Read the model definition and answer for the solid it produces. Units are mm, in the model's axes. Coordinates: 2 decimals unless noted, no trailing zeros. Order: outer loops, then holes, each group sorted by start corner. A loop starts at its lowest first (then second) coordinate and runs counter-clockwise, first axis right, second up.
```python
from build123d import *

# Parameters (mm, degrees)
SKETCH1_W           = 11.5
SKETCH1_H           = 11.5
BOSS_EXTRUDE1_DEPTH = 2
SKETCH2_R           = 2
CUT_EXTRUDE1_DEPTH  = 3
FILLET1_R           = 1
FILLET2_R           = 0.5
FILLET3_R           = 0.5


with BuildPart() as part:
    # Sketch1 → Boss-Extrude1 (new body)
    with BuildSketch(Plane(origin=(0, 0, 0), x_dir=(1, 0, 0), z_dir=(0, 1, 0))):
        Rectangle(SKETCH1_W, SKETCH1_H)
    extrude(amount=BOSS_EXTRUDE1_DEPTH)

    # Sketch2 → Cut-Extrude1 (cut, through all)
    with BuildSketch(Plane(origin=(0, 2, 0), x_dir=(1, 0, 0), z_dir=(0, 1, 0))):
        Circle(SKETCH2_R)
    extrude(amount=-CUT_EXTRUDE1_DEPTH, mode=Mode.SUBTRACT)

    # Fillet1
    fillet1_edges = [part.edges().sort_by_distance(p)[0] for p in [
        (0, 2, 5.75),
    ]]
    fillet(fillet1_edges, radius=FILLET1_R)

    # Fillet2
    fillet2_edges = [part.edges().sort_by_distance(p)[0] for p in [
        (0, 2, -5.75),
    ]]
    fillet(fillet2_edges, radius=FILLET2_R)

    # Fillet3
    fillet3_edges = [part.edges().sort_by_distance(p)[0] for p in [
        (-2, 2, 0),
    ]]
    fillet(fillet3_edges, radius=FILLET3_R)


solid = part.part
```
1) A cutting plane is placed at C-C, the plane y = 1.2. Determine the outline of the cut face in (x, z), and give its area (3 significant figures).
A:
outline: (-5.75, -5.75) - (5.75, -5.75) - (5.75, 5.73) - (-5.75, 5.73) - close; hole circle Ø4 at (0, 0)
area: 119 mm2
2) Straight lines are drawn through the part: line 1 (X direction, y = 0.3, z = 0); line 2 (X direction, y = 1.7, z = -1.75). For each, find the intervals that lie inside material, in ascending order.
A:
line 1: x = -5.75 to -2, 2 to 5.75
line 2: x = -5.75 to -1.05, 1.05 to 5.75
3) A cutting plane is placed at A-A, the plane z = 0. Determine the outline of the cut face in (x, y).
A:
outline: (-5.75, 0) - (-2, 0) - (-2, 1.5) arc R0.5 ccw to (-2.5, 2) - (-5.75, 2) - close; (2, 0) - (5.75, 0) - (5.75, 2) - (2.5, 2) arc R0.5 ccw to (2, 1.5) - close
4) A cutting plane is placed at B-B, the plane x = 0. Determine the outline of the cut face in (y, z), and give its area (3 significant figures).
A:
outline: (0, -5.75) - (1.5, -5.75) arc R0.5 ccw to (2, -5.25) - (2, -2.5) arc R0.5 ccw to (1.5, -2) - (0, -2) - close; (0, 2) - (1.5, 2) arc R0.5 ccw to (2, 2.5) - (2, 4.75) arc R1 ccw to (1, 5.75) - (0, 5.75) - close
area: 14.6 mm2
5) Flat-ended cylindrical pins translate along their axes: pin 1 Ø1.5 at (x, z) = (2.5, -2) entering from -Y; pin 2 Ø4.5 at (x, z) = (0, 0) entering from +Y. Find the tip coordinate at first contact, or state that the pin passes through.
A:
pin 1: stops at y = 0
pin 2: stops at y = 1.93
6) A cutting plane is placed at D-D, the plane z = 5.25. Determine the outline of the cut face in (x, y).
A:
outline: (-5.75, 0) - (5.75, 0) - (5.75, 1.87) - (-5.75, 1.87) - close
7) Determine the mould class of faces 1 (the flat face through (5.75, 1, 0)), 2 (the flat face through (-5.75, 1, 0)), 3 (the flat face through (-0.1, 0.5, 5.75)), 4 (the cylindrical face through (0, 1, 2)) for opening direction X: pulls with the +X half, pulls with the -X half, needs draft (parallel to the pull), parting line crosses it, or undercut.
A:
face 1: pulls with the +X half
face 2: pulls with the -X half
face 3: needs draft
face 4: undercut
